Here's how the part is built. I have some questions about the finished solid (model axes, mm). A direction names the side the tool comes from. Coordinates: 2 decimals unless noted, no trailing zeros. Order: outer loops, then holes, each group sorted by start corner. A loop starts at its lowest first (then second) coordinate and runs counter-clockwise, first axis right, second up. Notation, with made-up numbers: (69, 41.5) - (127, 41.5) arc R27 cw to (127, 75.5) - close; hole circle Ø11 at (-21, 26). An arc over 180 degrees is marked (long way). Use one line per item in the form item = value. Start each with the question number.
from build123d import *

# Parameters (mm, degrees)
SKETCH1_W           = 102.1
SKETCH1_H           = 147.765136106
SKETCH1_R           = 5.1
SKETCH1_R_2         = 3
SKETCH1_R_3         = 8.05
BOSS_EXTRUDE1_DEPTH = 3
BOSS_EXTRUDE2_DEPTH = 102.1
FILLET1_R           = 10
SKETCH3_R           = 8.05
BOSS_EXTRUDE3_DEPTH = 3
FILLET2_R           = 10


with BuildPart() as part:
    # Sketch1 → Boss-Extrude1 (new body)
    with BuildSketch(Plane.XY):
        with Locations((0, -22.832568053)):
            Rectangle(SKETCH1_W, SKETCH1_H)
        with Locations((-23, -63)):
            Circle(SKETCH1_R, mode=Mode.SUBTRACT)
        with Locations((2.86862691, -73.715136106)):
            Circle(SKETCH1_R_2, mode=Mode.SUBTRACT)
        with Locations((23, 23)):
            Circle(SKETCH1_R_3, mode=Mode.SUBTRACT)
        with Locations((0, -23)):
            Circle(SKETCH1_R_3, mode=Mode.SUBTRACT)
        with Locations((-23, -23)):
            Circle(SKETCH1_R_3, mode=Mode.SUBTRACT)
        Circle(SKETCH1_R_3, mode=Mode.SUBTRACT)
        with Locations((-23, 0)):
            Circle(SKETCH1_R_3, mode=Mode.SUBTRACT)
        with Locations((23, -23)):
            Circle(SKETCH1_R_3, mode=Mode.SUBTRACT)
        with Locations((23, 0)):
            Circle(SKETCH1_R_3, mode=Mode.SUBTRACT)
        with Locations((2.86862691, -52.284863894)):
            Circle(SKETCH1_R_2, mode=Mode.SUBTRACT)
        with Locations((0, 23)):
            Circle(SKETCH1_R_3, mode=Mode.SUBTRACT)
        with Locations((-23, 23)):
            Circle(SKETCH1_R_3, mode=Mode.SUBTRACT)
    extrude(amount=-BOSS_EXTRUDE1_DEPTH)

    # Sketch2 → Boss-Extrude2 (add)
    with BuildSketch(Plane.ZY.offset(51.05)):
        with BuildLine():
            Line((-24.480762114, -109.117059895), (-93.762794416, -69.117059895))
            Line((-93.762794416, -69.117059895), (-95.262794416, -71.715136106))
            Line((-95.262794416, -71.715136106), (-25.980762114, -111.715136106))
            ThreePointArc((-25.980762114, -111.715136106), (-8.660254038, -111.715136106), (0, -96.715136106))
            Line((0, -96.715136106), (-3, -96.715136106))
            ThreePointArc((-3, -96.715136106), (-10.160254038, -109.117059895), (-24.480762114, -109.117059895))
        make_face()
    extrude(amount=-BOSS_EXTRUDE2_DEPTH)

    # Fillet1
    fillet1_edges = [part.edges().sort_by_distance(p)[0] for p in [
        (51.05, 51.05, -1.5),
        (-51.05, 51.05, -1.5),
        (-51.05, -70.416098001, -94.512794416),
        (51.05, -70.416098001, -94.512794416),
    ]]
    fillet(fillet1_edges, radius=FILLET1_R)

    # Sketch3 → Boss-Extrude3 (add)
    with BuildSketch(Plane(origin=(0, 0, -3), x_dir=(-1, 0, 0), z_dir=(0, 0, -1))):
        with BuildLine():
            ThreePointArc((67.05, -81.715136106), (82.05, -66.715136106), (67.05, -51.715136106))
            Line((67.05, -51.715136106), (51.05, -51.715136106))
            Line((51.05, -51.715136106), (51.05, -81.715136106))
            Line((51.05, -81.715136106), (67.05, -81.715136106))
        make_face()
        with Locations((67.05, -66.715136106)):
            Circle(SKETCH3_R, mode=Mode.SUBTRACT)
    extrude(amount=-BOSS_EXTRUDE3_DEPTH)

    # Fillet2
    fillet2_edges = [part.edges().sort_by_distance(p)[0] for p in [
        (-51.05, -51.715136106, -1.5),
        (-51.05, -81.715136106, -1.5),
    ]]
    fillet(fillet2_edges, radius=FILLET2_R)


solid = part.part
1) Suppose I cut it at B-B, the plane y = -23. List the corners of the cut face in (x, z) for me.
2) Suppose I cut it at A-A, the plane x = -23. List the corners of the cut face in (y, z) for me.
3) Which directions (+Z, -Z, +X, -X, +Y, -Y) give clear straight access to the entire face, cutting with the end or side of a thin tool? Please do faces 1 (the flat face through (-0.715, -89.397, -58.637)), 2 (the cylindrical face through (2.48, -70.74, -1.48)), 3 (the flat face through (-51.05, -101, -40)), 4 (the cylindrical face through (-61.12, -61.27, -1.52)).
4) For pin 1 (2.5 mm diameter, centred on x = -65, z = -2, fed in from +Y); pin 2 (1.5 mm diameter, centred on x = -62.5, z = -2, fed in from -Y); pin 3 (1.5 mm diameter, centred on y = 16.5, z = -1, fed in from -X), each with a flat end and sliding along its axis, tell me the tip position at first contact or that it passes through.
5) Suppose I cut it at D-D, the plane y = -63. List the corners of the cut face in (x, z) for me.
6) I need wall thicknesses on probe 1 along Z at (x, y) = (-9, -59.5); probe 2 along Z at (x, y) = (-34, -92); probe 3 along Y at (x, z) = (26, -72). Which ranges of each line are inside material? Lowest first, please. Write a range as [from, to].
7) If we mould it in two halves opening along X, with no side actions, what happens to faces 5 (the cylindrical face through (48.2, 48.04, -1.52)), 6 (the cylindrical face through (-29.388, -27.898, -1.479)), 7 (the cylindrical face through (-53.902, -84.722, -1.479))? For each: pulls with the +X half, pulls with the -X half, needs draft (parallel to the pull), parting line crosses it, or undercut.
8) Suppose I cut it at C-C, the plane x = 22. List the corners of the cut face in (y, z) for me.
From the geometry:
q1.outline = (-51.05, -3) - (-31.05, -3) - (-31.05, 0) - (-51.05, 0) - close; (-14.95, -3) - (-8.05, -3) - (-8.05, 0) - (-14.95, 0) - close; (8.05, -3) - (14.95, -3) - (14.95, 0) - (8.05, 0) - close; (31.05, -3) - (51.05, -3) - (51.05, 0) - (31.05, 0) - close
q2.outline = (-111.72, -25.98) - (-71.72, -95.26) - (-69.12, -93.76) - (-109.12, -24.48) arc R14.32 cw to (-96.72, -3) - (-68.1, -3) - (-68.1, 0) - (-96.72, 0) arc R17.32 ccw to start; (-57.9, -3) - (-31.05, -3) - (-31.05, 0) - (-57.9, 0) - close; (-14.95, -3) - (-8.05, -3) - (-8.05, 0) - (-14.95, 0) - close; (8.05, -3) - (14.95, -3) - (14.95, 0) - (8.05, 0) - close; (31.05, -3) - (51.05, -3) - (51.05, 0) - (31.05, 0) - close
q3.face_1 = +X, -X, +Y
q3.face_2 = +Z
q3.face_3 = -Z, -X, -Y
q3.face_4 = +Z, -Z
q4.pin_1 = -51.72
q4.pin_2 = -81.72
q4.pin_3 = -51.05
q5.outline = (-81.58, -3) - (-74.19, -3) - (-74.19, 0) - (-81.58, 0) - close; (-59.91, -3) - (-28.1, -3) - (-28.1, 0) - (-59.91, 0) - close; (-17.9, -3) - (51.05, -3) - (51.05, 0) - (-17.9, 0) - close
q6.probe_1 = [-3, 0]
q6.probe_2 = [-60.13, -54.13], [-3, 0]
q6.probe_3 = [-85.15, -81.68]
q7.face_5 = pulls with the +X half
q7.face_6 = undercut
q7.face_7 = pulls with the -X half
q8.outline = (-111.72, -25.98) - (-71.72, -95.26) - (-69.12, -93.76) - (-109.12, -24.48) arc R14.32 cw to (-96.72, -3) - (-30.99, -3) - (-30.99, 0) - (-96.72, 0) arc R17.32 ccw to start; (-15.01, -3) - (-7.99, -3) - (-7.99, 0) - (-15.01, 0) - close; (7.99, -3) - (15.01, -3) - (15.01, 0) - (7.99, 0) - close; (30.99, -3) - (51.05, -3) - (51.05, 0) - (30.99, 0) - close
